Check sheet for the modelled part. Datum: model origin and axes. Units: mm. Give positions to 0.01 mm unless a question says otherwise; leave off trailing zeros. Write each loop counter-clockwise with the first axis right and the second up, starting at its lowest first coordinate (ties: lowest second). Pieces come first, ordered by that corner, then holes. Notation, with made-up numbers: (35, 37) -> (79, 37) arc R37 cw to (79, 75) -> close; hole circle Ø1 at (-40, 56). An arc over 180 degrees is marked (long way). Answer as a JSON object with one key per item and string values.
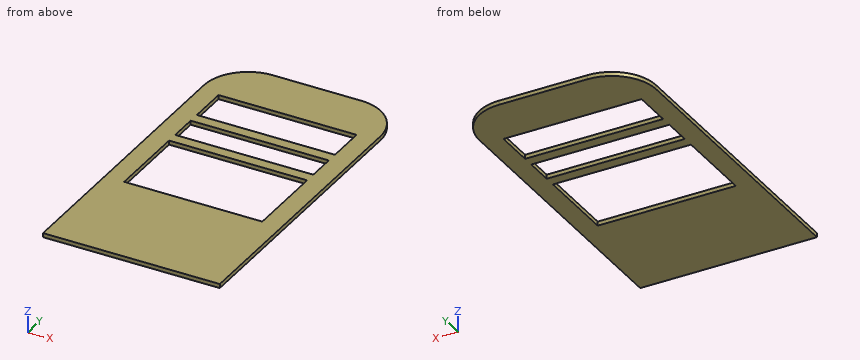
from build123d import *

# Parameters (mm, degrees)
F0_W     = 635
F0_H     = 126.999991
F0_H_2   = 177.800009
F1_DEPTH = 19.05


with BuildPart() as f1:
    # F0 (on Top) → F1 (new body)
    with BuildSketch(Plane.XY):
        with BuildLine():
            Line((-648.038619, 763.81958), (-648.038619, -556.98042))
            Line((-648.038619, -556.98042), (164.761381, -556.98042))
            Line((164.761381, -556.98042), (164.761381, 763.81958))
            ThreePointArc((164.761381, 763.81958), (105.245479, 907.503678), (-38.438619, 967.01958))
            Line((-38.438619, 967.01958), (-444.838619, 967.01958))
            ThreePointArc((-444.838619, 967.01958), (-588.522717, 907.503678), (-648.038619, 763.81958))
        make_face()
        Polygon((75.861381, -48.98042), (-559.138619, -48.98042), (-559.138619, 90.71958), (-559.138619, 141.51958), (-559.138619, 319.31958), (75.861381, 319.31958), (75.861381, 141.51958), (75.861381, 90.71958), align=None, mode=Mode.SUBTRACT)
        with Locations((-241.638619, 433.619575)):
            Rectangle(F0_W, F0_H, mode=Mode.SUBTRACT)
        with Locations((-241.638619, 636.819575)):
            Rectangle(F0_W, F0_H_2, mode=Mode.SUBTRACT)
    extrude(amount=F1_DEPTH)


solid = f1.part
1. Sectioned sample at D-D, the plane x = 49. Enter the section's corners in (y, z).
Determined:
{"outline": "(-556.98, 0) -> (-48.98, 0) -> (-48.98, 19.05) -> (-556.98, 19.05) -> close; (319.32, 0) -> (370.12, 0) -> (370.12, 19.05) -> (319.32, 19.05) -> close; (497.12, 0) -> (547.92, 0) -> (547.92, 19.05) -> (497.12, 19.05) -> close; (725.72, 0) -> (947.24, 0) -> (947.24, 19.05) -> (725.72, 19.05) -> close"}
2. Sectioned sample at A-A, the plane x = -206.5. Enter the section's corners in (y, z), plus the area to 3 significant figures.
Determined:
{"outline": "(-556.98, 0) -> (-48.98, 0) -> (-48.98, 19.05) -> (-556.98, 19.05) -> close; (319.32, 0) -> (370.12, 0) -> (370.12, 19.05) -> (319.32, 19.05) -> close; (497.12, 0) -> (547.92, 0) -> (547.92, 19.05) -> (497.12, 19.05) -> close; (725.72, 0) -> (967.02, 0) -> (967.02, 19.05) -> (725.72, 19.05) -> close", "area": "16,200 mm^2"}
3. Go/stop test with a flat-tipped pin: P1, Ø3, axis at x = -423.5, y = 723.5, coming from the +Z side. Record where the tip stops, or that it passes through.
Determined:
{"P1": "through"}
4. Sectioned sample at C-C, the plane z = 7.25. Enter the section's corners in (x, y), plus the area to 3 significant figures.
Determined:
{"outline": "(-648.04, -556.98) -> (164.76, -556.98) -> (164.76, 763.82) arc R203.2 ccw to (-38.44, 967.02) -> (-444.84, 967.02) arc R203.2 ccw to (-648.04, 763.82) -> close; hole (-559.14, -48.98) -> (75.86, -48.98) -> (75.86, 319.32) -> (-559.14, 319.32) -> close; hole (-559.14, 370.12) -> (75.86, 370.12) -> (75.86, 497.12) -> (-559.14, 497.12) -> close; hole (-559.14, 547.92) -> (75.86, 547.92) -> (75.86, 725.72) -> (-559.14, 725.72) -> close", "area": "794,000 mm^2"}
5. Scan lines: L1, parallel to Y at x = -380.5, z = 13.75; L2, parallel to X at y = 457, z = 17.5; L3, parallel to Y at x = -501, z = 15.5. Record each from-to range of solid material in increasing order. Write a range as [from, to].
Determined:
{"L1": "[-556.98, -48.98], [319.32, 370.12], [497.12, 547.92], [725.72, 967.02]", "L2": "[-648.04, -559.14], [75.86, 164.76]", "L3": "[-556.98, -48.98], [319.32, 370.12], [497.12, 547.92], [725.72, 959.1]"}
6. Sectioned sample at B-B, the plane y = 225.5. Enter the section's corners in (x, z), plus the area to 3 significant figures.
Determined:
{"outline": "(-648.04, 0) -> (-559.14, 0) -> (-559.14, 19.05) -> (-648.04, 19.05) -> close; (75.86, 0) -> (164.76, 0) -> (164.76, 19.05) -> (75.86, 19.05) -> close", "area": "3,390 mm^2"}
